Input: dimensioned drawing with shaded views. Units: mm. Origin: part minimum x, y, z. A direction names the side the tool comes from. Round coordinates to 2 decimals unless told otherwise and drop trailing zeros. Order: outer loops, then holes, each group sorted by start corner. A loop starts at its lowest first (then second) coordinate and runs counter-clockwise, first axis right, second up.
Item 1: First-contact query: pin 1 (2.5 mm diameter, centred on x = 31, y = 5, fed in from +Z); pin 2 (1.8 mm diameter, centred on x = 4.6, y = 30.6, fed in from +Z); pin 3 (1 mm diameter, centred on x = 15.5, y = 11, fed in from +Z). Flat tips, straight axial feed; report the tip coordinate or a pass-through.
Item 2: Reachability of the marked faces 1 and 2 from +Z, -Z, +X, -X, +Y, -Y: full face, straight path, thin tool, end or side. Return the list, or none.
Item 3: Cut plane B-B on y = 4.6. Output: boundary loops of the cut face in (x, z), then the cut area to 3 significant figures.
Item 4: Line query: L1, parallel to Y at x = 30.6, z = 48.25; L2, parallel to X at y = 30, z = 47. Output: solid intervals per line, ascending.
Item 5: Cut plane C-C on x = 9. Output: boundary loops of the cut face in (y, z), then the cut area to 3 significant figures.
Item 6: Cut plane A-A on z = 44.5. Output: boundary loops of the cut face in (x, y), then the cut area to 3 significant figures.
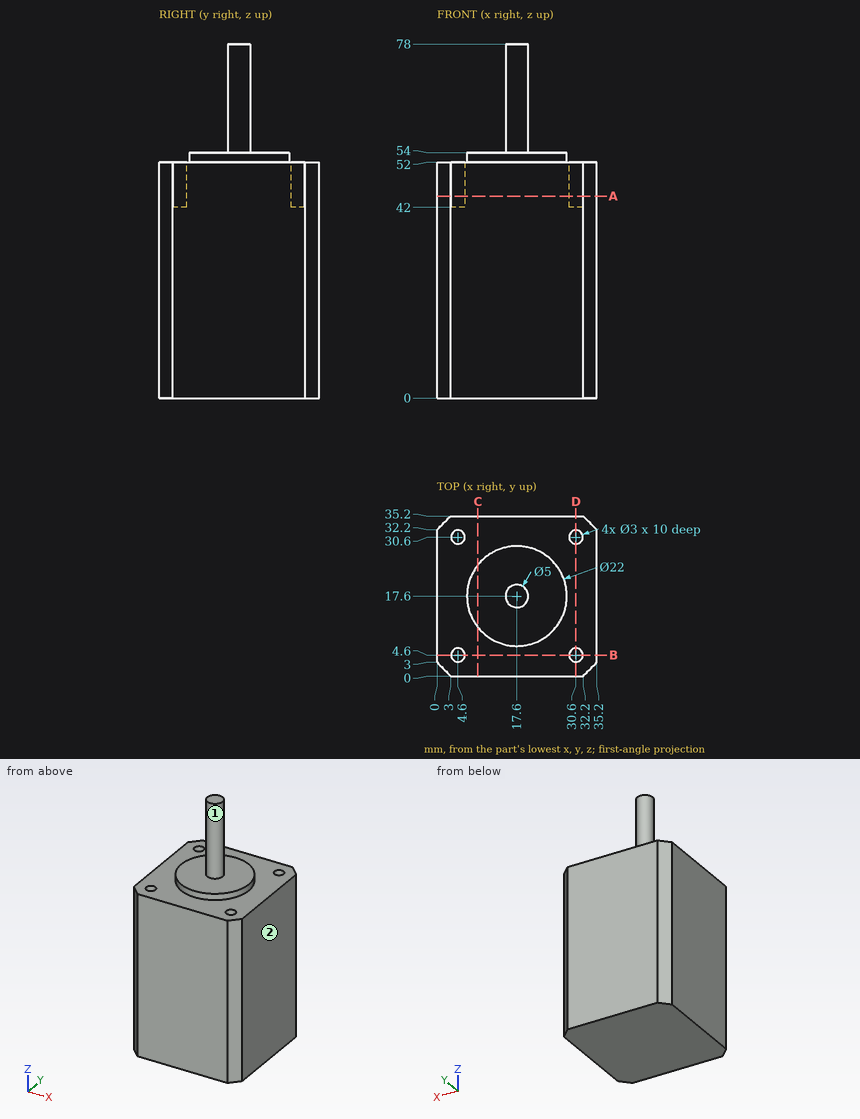
From the geometry:
1. pin 1: stops at z = 52
1. pin 2: stops at z = 42
1. pin 3: stops at z = 54
2. face 1: +Z
2. face 2: +Z, -Z, +X, +Y, -Y
3. outline: (0, 0) - (35.2, 0) - (35.2, 52) - (32.1, 52) - (32.1, 42) - (29.1, 42) - (29.1, 52) - (6.1, 52) - (6.1, 42) - (3.1, 42) - (3.1, 52) - (0, 52) - close
3. area: 1,770 mm2
4. L1: y = 0 to 3.1, 6.1 to 29.1, 32.1 to 35.2
4. L2: x = 0 to 3.23, 5.97 to 29.23, 31.97 to 35.2
5. outline: (0, 0) - (35.2, 0) - (35.2, 52) - (24.46, 52) - (24.46, 54) - (10.74, 54) - (10.74, 52) - (0, 52) - close
5. area: 1,860 mm2
6. outline: (0, 3) - (3, 0) - (32.2, 0) - (35.2, 3) - (35.2, 32.2) - (32.2, 35.2) - (3, 35.2) - (0, 32.2) - close; hole circle Ø3 at (4.6, 4.6); hole circle Ø3 at (4.6, 30.6); hole circle Ø3 at (30.6, 4.6); hole circle Ø3 at (30.6, 30.6)
6. area: 1,190 mm2
